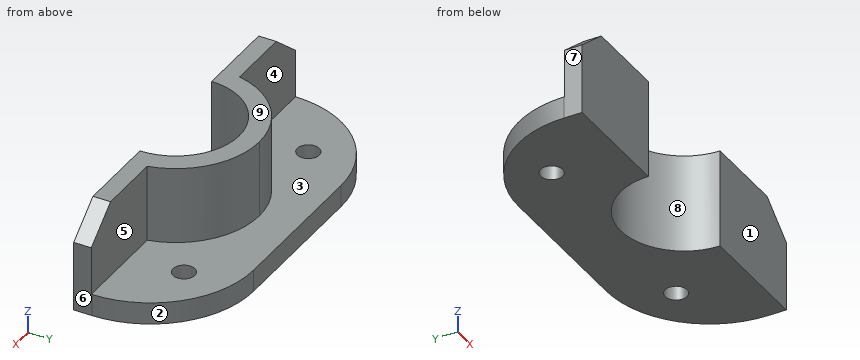
from build123d import *

# Parameters (mm, degrees)
ESTRUSIONE_ESTRUSIONE1_DEPTH = 20
ESTRUSIONE_ESTRUSIONE3_DEPTH = 5
RACCORDO1_R                  = 47
SCHIZZO5_R                   = 5
TAGLIO_ESTRUSIONE1_DEPTH     = 10
TAGLIO_ESTRUSIONE2_DEPTH     = 10
RACCORDO1_OF_SPECCHIA2_R     = 47


with BuildPart() as part:
    # Schizzo1 → Estrusione-Estrusione1 (new body, symmetric)
    with BuildSketch(Plane.XY):
        with BuildLine():
            Line((28.869072897, 0), (82.088181758, 0))
            Line((82.088181758, 0), (82.088181758, 8))
            Line((82.088181758, 8), (37.134650395, 8))
            ThreePointArc((37.134650395, 8), (23.865135757, 29.553976979), (0, 37.986606324))
            Line((0, 37.986606324), (0, 28.869072897))
            ThreePointArc((0, 28.869072897), (20.413517212, 20.413517212), (28.869072897, 0))
        make_face()
    estrusione_estrusione1 = extrude(amount=ESTRUSIONE_ESTRUSIONE1_DEPTH, both=True)

    # Schizzo4 → Estrusione-Estrusione3 (add, symmetric)
    with BuildSketch(Plane(origin=(0, 0, -20), x_dir=(-1, 0, 0), z_dir=(0, 0, -1))):
        with BuildLine():
            Line((-28.869072897, 0), (-82.088181758, 0))
            Line((-82.088181758, 0), (-82.088181758, 55.326384445))
            Line((-82.088181758, 55.326384445), (0, 55.326384445))
            Line((0, 55.326384445), (0, 28.869072897))
            ThreePointArc((0, 28.869072897), (-20.413517212, 20.413517212), (-28.869072897, 0))
        make_face()
    estrusione_estrusione3 = extrude(amount=ESTRUSIONE_ESTRUSIONE3_DEPTH, both=True)

    # Raccordo1
    raccordo1_edges = [part.edges().sort_by_distance(p)[0] for p in [
        (82.088181758, 55.326384445, -20),
    ]]
    fillet(raccordo1_edges, radius=RACCORDO1_R)

    # Schizzo5 → Taglio-Estrusione1 (cut)
    with BuildSketch(Plane.XY.offset(-15)):
        with Locations((50, 32)):
            Circle(SCHIZZO5_R)
    taglio_estrusione1 = extrude(amount=-TAGLIO_ESTRUSIONE1_DEPTH, mode=Mode.SUBTRACT)

    # Schizzo6 → Taglio-Estrusione2 (cut)
    with BuildSketch(Plane(origin=(0, 8, 0), x_dir=(1, 0, 0), z_dir=(0, 1, 0))):
        Polygon((66.595385054, -20), (82.088181758, -7), (82.088181758, -20), align=None)
    taglio_estrusione2 = extrude(amount=-TAGLIO_ESTRUSIONE2_DEPTH, mode=Mode.SUBTRACT)

    # Specchia2: Estrusione-Estrusione1, Estrusione-Estrusione3, Taglio-Estrusione1, Taglio-Estrusione2 across plane
    add(estrusione_estrusione1.mirror(Plane(origin=(0, 0, 0), x_dir=(0, 0, 1), z_dir=(1, 0, 0))))
    add(estrusione_estrusione3.mirror(Plane(origin=(0, 0, 0), x_dir=(0, 0, 1), z_dir=(1, 0, 0))))
    add(taglio_estrusione1.mirror(Plane(origin=(0, 0, 0), x_dir=(0, 0, 1), z_dir=(1, 0, 0))), mode=Mode.SUBTRACT)
    add(taglio_estrusione2.mirror(Plane(origin=(0, 0, 0), x_dir=(0, 0, 1), z_dir=(1, 0, 0))), mode=Mode.SUBTRACT)

    # Raccordo1 of Specchia2
    raccordo1_of_specchia2_edges = [part.edges().sort_by_distance(p)[0] for p in [
        (-82.088181758, 55.326384445, -20),
    ]]
    fillet(raccordo1_of_specchia2_edges, radius=RACCORDO1_OF_SPECCHIA2_R)


solid = part.part
Work out the finished part from the listing and answer in its coordinate system (mm). Face numbers are marked on the shaded views. A direction names the side the tool comes from. Coordinates: 2 decimals unless noted, no trailing zeros. Order: outer loops, then holes, each group sorted by start corner. A loop starts at its lowest first (then second) coordinate and runs counter-clockwise, first axis right, second up. Notation, with made-up numbers: (60, -26.5) - (94, -26.5) arc R28 ccw to (94, -2.5) - close; hole circle Ø4 at (-31.5, 40.25). An arc over 180 degrees is marked (long way). Put each result on its own line as item: value. Start each with the question number.
1) Find section D-D (z = -3). Give the vertices of the cut face in (x, y), plus the area to 3 significant figures.
2) For the marked faces 1, 2, 3, 4 and 5, determine the directions among +Z, -Z, +X, -X, +Y, -Y from which every point of the face is accessible in a straight line to the end or side of a thin tool.
3) Find section C-C (y = 23). Give the vertices of the cut face in (x, z), plus the area to 3 significant figures.
4) Find the intervals of material crossed by line 1 (Y direction, x = -59.5, z = 16.5); line 2 (Z direction, x = 39.5, y = 42); line 3 (Y direction, x = -50, z = -19), in increasing order. Write a range as from..to.
5) Find section B-B (x = 50). Give the vertices of the cut face in (y, z), plus the area to 3 significant figures.
6) Flat-ended cylindrical pins translate along their axes: pin 1 (5 mm diameter, centred on x = 56, y = 12, fed in from +Z); pin 2 (8 mm diameter, centred on x = -50, y = 32, fed in from +Z); pin 3 (14 mm diameter, centred on x = -18.5, y = 40.5, fed in from +Z); pin 4 (6 mm diameter, centred on y = 24, z = 14.5, fed in from -X). Find the tip coordinate at first contact, or state that the pin passes through.
7) Find section A-A (z = -21). Give the vertices of the cut face in (x, y), plus the area to 3 significant figures.
8) For a pull along X with two mould halves and no side action, classify the marked faces 6, 7, 8 and 9 as released by +X, released by -X, zero draft, split by the parting line, or undercut.
Results list:
1. outline: (-82.09, 0) - (-28.87, 0) arc R28.87 cw to (28.87, 0) - (82.09, 0) - (82.09, 8) - (37.13, 8) arc R37.99 ccw to (-37.13, 8) - (-82.09, 8) - close
1. area: 1,670 mm^2
2. face 1: +Z, -Z, +X, -X, -Y
2. face 2: +Z, -Z, +X, +Y
2. face 3: +Z, +Y
2. face 4: +Z, -X, +Y
2. face 5: +Z, +X, +Y
3. outline: (-79.74, -25) - (-17.45, -25) - (-17.45, 20) - (-30.23, 20) - (-30.23, -15) - (-79.74, -15) - close; (17.45, -25) - (79.74, -25) - (79.74, -15) - (30.23, -15) - (30.23, 20) - (17.45, 20) - close
3. area: 2,140 mm^2
4. line 1: y = 0..8
4. line 2: z = -25..-15
4. line 3: y = 0..27, 37..52.9
5. outline: (0, -25) - (27, -25) - (27, -15) - (8, -15) - (8, 20) - (0, 20) - close; (37, -25) - (52.9, -25) - (52.9, -15) - (37, -15) - close
5. area: 709 mm^2
6. pin 1: stops at z = -15
6. pin 2: passes through
6. pin 3: stops at z = 20
6. pin 4: stops at x = -31.65
7. outline: (-82.09, 0) - (-28.87, 0) arc R28.87 cw to (28.87, 0) - (82.09, 0) - (82.09, 8.33) arc R47 ccw to (35.09, 55.33) - (-35.09, 55.33) arc R47 ccw to (-82.09, 8.33) - close; hole circle Ø10 at (-50, 32); hole circle Ø10 at (50, 32)
7. area: 6,670 mm^2
8. face 6: released by +X
8. face 7: released by -X
8. face 8: undercut
8. face 9: zero draft
